The model under review builds one solid part; all positions refer to its coordinate system, in mm. A direction names the side the tool comes from. Coordinates: 2 decimals unless noted, no trailing zeros. Loops run counter-clockwise (first coordinate to the right, second up) from the corner with the lowest first, then second, coordinate; pieces in that order, holes last. Notation, with made-up numbers: M -1.5,75.25 L 6.5,75.25 A17 cw 6.5,95.25 Z; hole C 46.25,73.25 d11. An arc over 180 degrees is marked long. Use one line per item in the form item = value.
```python
from build123d import *

# Parameters (mm, degrees)
SKETCH_1_W          = 125
SKETCH_1_H          = 60
EXTRUDE_1_DEPTH     = 6
FILLET_1_R          = 10
CUT_EXTRUDE_1_DEPTH = 4
CHAMFER_1_SIZE      = 2
SKETCH_4_W          = 118
SKETCH_4_H          = 1.5
EXTRUDE_3_DEPTH     = 4
SKETCH_3_R          = 1
CUT_EXTRUDE_2_DEPTH = 10
SKETCH_5_R          = 1
CUT_EXTRUDE_3_DEPTH = 10
SKETCH_6_R          = 10
CUT_EXTRUDE_4_DEPTH = 2
CHAMFER_2_SIZE      = 0.5


with BuildPart() as part:
    # Эскиз1 → Бобышка-Вытянуть1 (new body)
    with BuildSketch(Plane(origin=(0, 0, 0), x_dir=(1, 0, 0), z_dir=(0, 1, 0))):
        Rectangle(SKETCH_1_W, SKETCH_1_H)
    extrude(amount=EXTRUDE_1_DEPTH)

    # Скругление1
    fillet_1_edges = [part.edges().sort_by_distance(p)[0] for p in [
        (62.5, 3, 30),
        (-62.5, 3, 30),
    ]]
    fillet(fillet_1_edges, radius=FILLET_1_R)

    # Эскиз2 → Вырез-Вытянуть1 (cut)
    with BuildSketch(Plane.XZ):
        with BuildLine():
            Line((-59, 20), (-59, -26.5))
            Line((-59, -26.5), (59, -26.5))
            Line((59, -26.5), (59, 20))
            ThreePointArc((59, 20), (57.096194078, 24.596194078), (52.5, 26.5))
            Line((52.5, 26.5), (-52.5, 26.5))
            ThreePointArc((-52.5, 26.5), (-57.096194078, 24.596194078), (-59, 20))
        make_face()
    extrude(amount=-CUT_EXTRUDE_1_DEPTH, mode=Mode.SUBTRACT)

    # Фаска1
    chamfer_1_edges = [part.edges().sort_by_distance(p)[0] for p in [
        (0, 0, 30),
        (62.5, 0, -5),
        (59.571067812, 0, 27.071067812),
        (-59.571067812, 0, 27.071067812),
        (-62.5, 0, -5),
        (0, 0, -30),
    ]]
    chamfer(chamfer_1_edges, length=CHAMFER_1_SIZE)

    # Эскиз4 → Бобышка-Вытянуть3 (add)
    with BuildSketch(Plane.XZ.offset(-4)):
        with Locations((0, -25.75)):
            Rectangle(SKETCH_4_W, SKETCH_4_H)
    extrude(amount=EXTRUDE_3_DEPTH)

    # Эскиз3 → Вырез-Вытянуть2 (cut)
    with BuildSketch(Plane(origin=(62.5, 0, 0), x_dir=(0, 0, -1), z_dir=(1, 0, 0))):
        with Locations((28, 4)):
            Circle(SKETCH_3_R)
    extrude(amount=-CUT_EXTRUDE_2_DEPTH, mode=Mode.SUBTRACT)

    # Эскиз5 → Вырез-Вытянуть3 (cut)
    with BuildSketch(Plane.ZY.offset(62.5)):
        with Locations((-28, 4)):
            Circle(SKETCH_5_R)
    extrude(amount=-CUT_EXTRUDE_3_DEPTH, mode=Mode.SUBTRACT)

    # Эскиз6 → Вырез-Вытянуть4 (cut)
    with BuildSketch(Plane.XZ.offset(-4)):
        with Locations((0, 12.5)):
            Circle(SKETCH_6_R)
    extrude(amount=-CUT_EXTRUDE_4_DEPTH, mode=Mode.SUBTRACT)

    # Фаска2
    chamfer_2_edges = [part.edges().sort_by_distance(p)[0] for p in [
        (0, 6, -30),
        (-10, 4, 12.5),
        (-10, 6, 12.5),
    ]]
    chamfer(chamfer_2_edges, length=CHAMFER_2_SIZE)


solid = part.part
```
1. Add section C-C (z = 12.5). State the section outline as (x, y) points, then the cut area to 4 significant figures.
Response values:
outline = M -62.5,2 L -60.5,0 L -59,0 L -59,4 L -10.5,4 L -10,4.5 L -10,5.5 L -10.5,6 L -62.5,6 Z; M 10,4.5 L 10.5,4 L 59,4 L 59,0 L 60.5,0 L 62.5,2 L 62.5,6 L 10.5,6 L 10,5.5 Z
area = 233.5 mm^2
2. Insertion check: P1, Ø1.8, axis at y = 4, z = -28, coming from the +X side; P2, Ø1.2, axis at y = 4, z = -28, coming from the -X side; P3, Ø15.5, axis at x = 26, z = 1.5, coming from the -Y side; P4, Ø1.6, axis at y = 4.5, z = -28, coming from the +X side. Each pin has a flat end and moves straight along its axis. Give the tip position at first contact, or say it passes through.
Response values:
P1 = 52.5
P2 = -52.5
P3 = 4
P4 = 62.5
3. Add section B-B (x = 0). State the section outline as (y, z) points, then the cut area to 3 significant figures.
Response values:
outline = M 0,-28 L 2,-30 L 5.5,-30 L 6,-29.5 L 6,2 L 5.5,2.5 L 4.5,2.5 L 4,2 L 4,-25 L 0,-25 Z; M 0,26.5 L 4,26.5 L 4,23 L 4.5,22.5 L 5.5,22.5 L 6,23 L 6,30 L 2,30 L 0,28 Z
area = 109 mm^2
4. Machinability: for faces 1 (the face through (-59, 2, -2)), 2 (the face through (59.49, 4.03, 27.15)), which of the approach directions +Z, -Z, +X, -X, +Y, -Y give a long, thin tool a straight path to every point of the face, cutting with its end or side? Answer none if there is none.
Response values:
face_1 = -Y
face_2 = +Z, +X, +Y, -Y
5. Add section D-D (z = -7.5). State the section outline as (x, y) points, then the cut area to 3 significant figures.
Response values:
outline = M -62.5,2 L -60.5,0 L -59,0 L -59,4 L 59,4 L 59,0 L 60.5,0 L 62.5,2 L 62.5,6 L -62.5,6 Z
area = 274 mm^2
6. The part is to be moulded in two halves that separate along Z. For faces 3 (the face through (-1, 2, -25)), 4 (the face through (-58.63, 0.57, 25.99)), 5 (the face through (62.5, 4, -5)), say which applies: pulls with the +Z half, pulls with the -Z half, needs draft (parallel to the pull), parting line crosses it, or undercut.
Response values:
face_3 = undercut
face_4 = pulls with the +Z half
face_5 = needs draft
7. Wall thickness on line 1 along Y through (x, z) = (-58.25, -28); line 2 along X through (y, z) = (2.5, 2); line 3 along Y through (x, z) = (-17.5, -18): over which ranges is each line inside the solid? List them lowest first. Write a range as from..to.
Response values:
line_1 = 0..3, 5..6
line_2 = -62.5..-59, 59..62.5
line_3 = 4..6
8. Add section A-A (y = 1). State the section outline as (x, z) points.
Response values:
outline = M -61.5,-29 L 61.5,-29 L 61.5,20 A9 ccw 52.5,29 L -52.5,29 A9 ccw -61.5,20 Z; hole M -59,-25 L 59,-25 L 59,20 A6.5 ccw 52.5,26.5 L -52.5,26.5 A6.5 ccw -59,20 Z
